Can you work these out from the drawing? Everything is in mm from the part's minimum corner. Give positions to 0.01 mm unless a question says otherwise; leave off trailing zeros. Write each loop counter-clockwise with the first axis right and the second up, starting at its lowest first coordinate (ties: lowest second). Pieces come first, ordered by that corner, then holes. Notation, with made-up numbers: (-12, 21) - (1, 21) arc R8 ccw to (1, 36) - close; hole circle Ø7 at (85, -24.75). An arc over 180 degrees is marked (long way). Write each question's results on one line, items separated by ' | '. Start each with the question number.
Item 1: Will these pins go through, and if not, where does the flat tip stop? P1, Ø1.5, axis at y = 28.5, z = 3.5, coming from the -X side; P2, Ø1.2, axis at x = 23.5, z = 3, coming from the +Y side; P3, Ø2.5, axis at y = 338, z = 2.5, coming from the +X side.
Item 2: Please list where these lines run through material, in increasing order: line 1 along Y through (x, z) = (12.5, 1.5); line 2 along Y through (x, z) = (10.75, 2); line 3 along X through (y, z) = (175, 1.1).
Item 3: Suppose I cut it at A-A on z = 4.2. List the corners of the cut face in (x, y) for me.
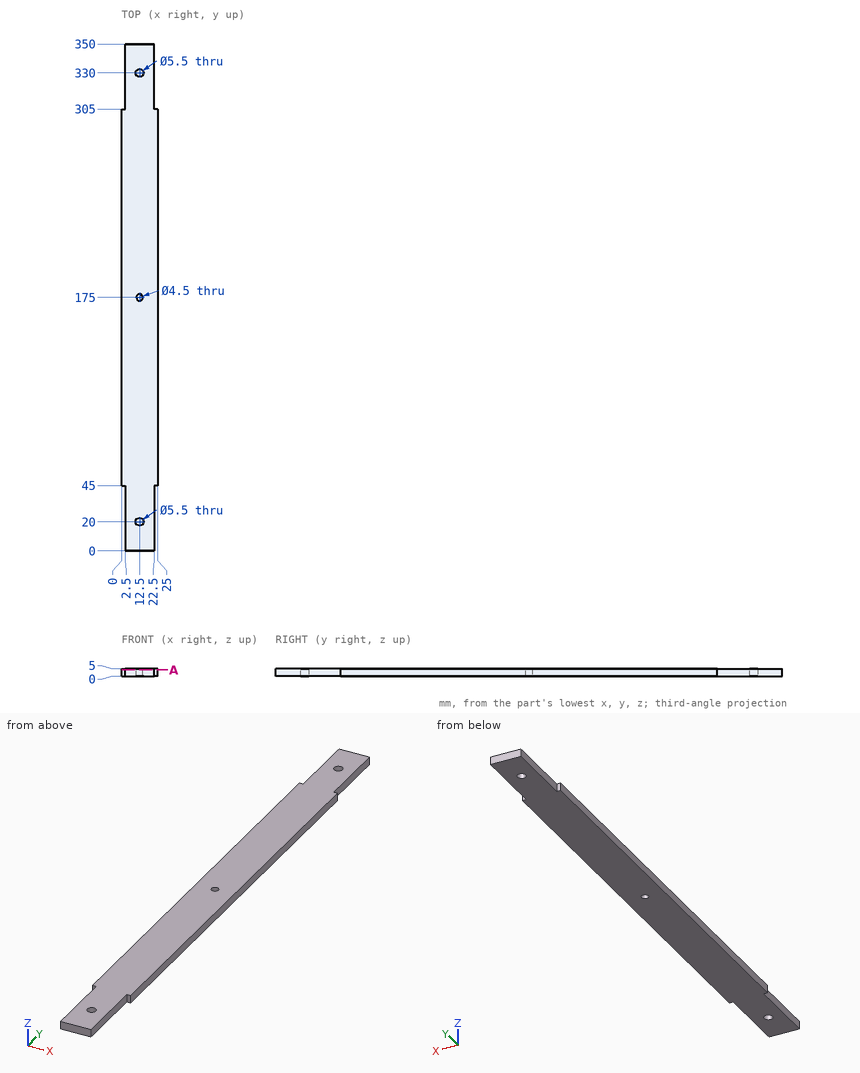
Checked values:
1) P1: stops at x = 2.5 | P2: stops at y = 305 | P3: stops at x = 22.5
2) line 1: y = 0 to 17.25, 22.75 to 172.75, 177.25 to 327.25, 332.75 to 350 | line 2: y = 0 to 17.88, 22.12 to 173.59, 176.41 to 327.88, 332.12 to 350 | line 3: x = 0 to 10.25, 14.75 to 25
3) outline: (0, 45) - (2.5, 45) - (2.5, 0) - (22.5, 0) - (22.5, 45) - (25, 45) - (25, 305) - (22.5, 305) - (22.5, 350) - (2.5, 350) - (2.5, 305) - (0, 305) - close; hole circle Ø5.5 at (12.5, 20); hole circle Ø5.5 at (12.5, 330); hole circle Ø4.5 at (12.5, 175)
